Autodesk Inventor part; units mm, degrees
ref_plane "YZ Plane" through (0, 0, 0) normal (1, 0, 0) x (0, 1, 0)
ref_plane "XZ Plane" through (0, 0, 0) normal (0, 1, 0) x (-1, 0, 0)
ref_plane "XY Plane" through (0, 0, 0) normal (0, 0, 1) x (1, 0, 0)
sketch "Sketch1" plane through (0, 0, 0) normal (0, 1, 0) x (-1, 0, 0)
  arc A0 (-3.9799, 0.4) -> (3.9799, 0.4) centre (0, 0) ccw
  line L0 (-3.9799, 0.4) -> (0, 40)
  line L1 (0, 40) -> (3.9799, 0.4)
  dimension "d0" = 4
  dimension "d1" = 40
sketch "Sketch2" plane through (0, 0, 0) normal (1, 0, 0) x (0, 1, 0)
  line L0 (0, 0) -> (-90, 60)
  dimension "d2" = 90
  dimension "d3" = 60
sweep "Sweep1" add profiles "Sketch1" path "Sketch2"
sketch "Sketch3" plane through (0, 0, 0) normal (0, 1, 0) x (1, 0, 0)
  circle A0 centre (0, 0) radius 3.5
  dimension "d6" = 7
extrude "Extrusion1" add sketch "Sketch3" along normal blind 204
sketch "Sketch4" plane through (0, 204, 0) normal (0, 1, 0) x (1, 0, 0)
  circle A0 centre (0, 0) radius 3
  circle A1 centre (0, 0) radius 5
  line L0 (-0.5, -5) -> (0.5, -5)
  line L1 (0.5, -5) -> (0.5, 5)
  line L2 (0.5, 5) -> (-0.5, 5)
  line L3 (-0.5, 5) -> (-0.5, -5)
  line L4 (-0.5, -5) -> (0.5, 5) construction
  line L5 (0.5, -5) -> (-0.5, 5) construction
  point P0 (-0.5, -2.958)
  point P1 (-0.5, 2.958)
  point P2 (0.5, 2.958)
  point P3 (0.5, -2.958)
  dimension "d9" = 6
  dimension "d10" = 10
  dimension "d11" = 1
  dimension "d12" = 10
extrude "Extrusion2" cut sketch "Sketch4" against normal blind 10 contours A0 L1 A1 | L1 A0 L3 | A0 L3 A1 L1 | L1 A1 L3 A0 | A0 L3 A1
thread "Thread1"
properties part number "rudder_pair_queens"
Design review of the part built by this model. Coordinates are the model's own, in mm. A direction names the side the tool comes from. Give positions to 0.01 mm unless a question says otherwise; leave off trailing zeros. Write each loop counter-clockwise with the first axis right and the second up, starting at its lowest first coordinate (ties: lowest second). Pieces come first, ordered by that corner, then holes.
(1) Tool access review of faces 1 (the face through (-3, 199, 0)), 2 (the face through (3, 199, 0)), 3 (the face through (0.5, 199, 0)), 4 (the face through (1.96, -45.63, 50.9)): name each direction out of +Z, -Z, +X, -X, +Y, -Y from which nothing blocks a thin tool from reaching the whole face with its end or side.
Checked values:
face 1: -X, +Y
face 2: +X, +Y
face 3: +Z, -Z, +Y
face 4: +Z, +X, +Y
(2) Clearance check with flat-ended pins moving along their axes: pin 1 Ø6.5 at (y, z) = (198.5, 0.5) entering from +X; pin 2 Ø3 at (y, z) = (196.5, 0) entering from -X; pin 3 Ø2 at (x, y) = (1.5, 103.5) entering from +Z. State where each tip first meets the part, or that it passes through.
Checked values:
pin 1: stops at x = 3
pin 2: stops at x = -3
pin 3: stops at z = 3.46
(3) Add section A-A (z = 80). Give the boundary of the cut face in (x, y), and give its area (3 significant figures).
Checked values:
outline: (-2.01, -90) - (2.01, -90) - (0, -60) - close
area: 60.3 mm2
(4) Wall thickness on line 1 along Z through (x, y) = (-1.75, 108.5); line 2 along X through (y, z) = (-63.5, 77); line 3 along Z through (x, y) = (1.5, 137.5): over which ranges is each line inside the solid? List them lowest first.
Checked values:
line 1: z = -3.03 to 3.03
line 2: x = -0.54 to 0.54
line 3: z = -3.16 to 3.16
(5) Mouldability with a two-part tool opening along X and no side actions: class faces 5 (the face through (-0.5, 199, 0)), 6 (the face through (0, 0, 13)), 7 (the face through (-2.1, -45.6, 49.5)), 8 (the face through (3.233, 95.642, -1.341)) as +X half, -X half, draft (parallel to the pull), parting line (faces both ways), or undercut.
Checked values:
face 5: undercut
face 6: draft
face 7: -X half
face 8: parting line
